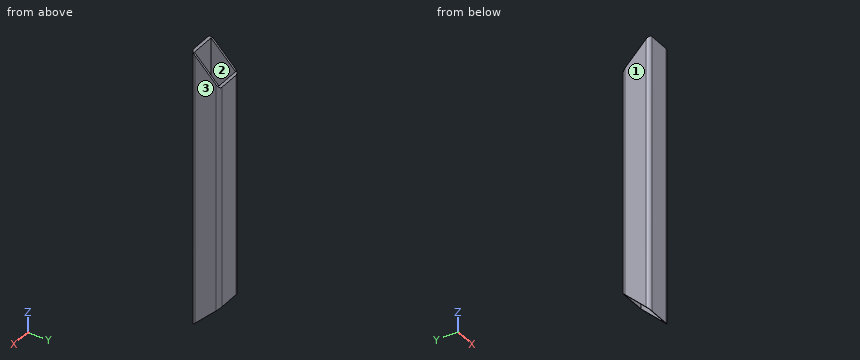
```python
from build123d import *

# Parameters (mm, degrees)
SKETCH1_W           = 50.8
SKETCH1_H           = 50.8
SKETCH1_W_2         = 44.45
SKETCH1_H_2         = 44.45
BOSS_EXTRUDE1_DEPTH = 254
FILLET1_R           = 6.35
CUT_EXTRUDE1_DEPTH  = 914.4


with BuildPart() as part:
    # Sketch1 → Boss-Extrude1 (new, symmetric)
    with BuildSketch(Plane.XY):
        Rectangle(SKETCH1_W, SKETCH1_H)
        Rectangle(SKETCH1_W_2, SKETCH1_H_2, mode=Mode.SUBTRACT)
    extrude(amount=BOSS_EXTRUDE1_DEPTH, both=True)

    # Fillet1
    fillet1_edges = [part.edges().sort_by_distance(p)[0] for p in [
        (-25.4, 25.4, 0),
        (25.4, 25.4, 0),
        (25.4, -25.4, 0),
        (-25.4, -25.4, 0),
    ]]
    fillet(fillet1_edges, radius=FILLET1_R)

    # Sketch2 → Cut-Extrude1 (cut)
    with BuildSketch(Plane.ZY.offset(25.4)):
        Polygon((254, -25.4), (203.2, 25.4), (254, 25.4), align=None)
        Polygon((-254, 25.4), (-254, -25.4), (-203.2, 25.4), align=None)
    extrude(amount=-CUT_EXTRUDE1_DEPTH, mode=Mode.SUBTRACT)


solid = part.part
```
Input: part model. Units: mm. Frame: model coordinates. Face numbers are marked on the shaded views. Give positions to 0.01 mm unless a question says otherwise; leave off trailing zeros. Order: outer loops, then holes, each group sorted by start corner. A loop starts at its lowest first (then second) coordinate and runs counter-clockwise, first axis right, second up. Notation, with made-up numbers: M 63,28.5 L 115,28.5 A22 cw 115,58.5 Z; hole C 12,-22.5 d9. An arc over 180 degrees is marked long. Return JSON: item names as keys, results as strings.
Item 1: Cut plane B-B (x = 9). Return loops of the section in (y, z) (3 decimals).
Solutions:
{"outline": "M -25.4,-254 L -22.225,-250.825 L -22.225,250.825 L -25.4,254 Z; M 22.225,-206.375 L 25.4,-203.2 L 25.4,203.2 L 22.225,206.375 Z"}
Item 2: Cut plane C-C (z = 49). Return loops of the section in (x, y) (3 decimals).
Solutions:
{"outline": "M -25.4,-19.05 A6.35 ccw -19.05,-25.4 L 19.05,-25.4 A6.35 ccw 25.4,-19.05 L 25.4,19.05 A6.35 ccw 19.05,25.4 L -19.05,25.4 A6.35 ccw -25.4,19.05 Z; hole M -22.225,-22.225 L 22.225,-22.225 L 22.225,22.225 L -22.225,22.225 Z"}
Item 3: Ray query, probe 1 along X at (y, z) = (-16.5, 126) (3 decimals); probe 2 along X at (y, z) = (-20, -231) (3 decimals); probe 3 along Y at (x, z) = (19.5, -142.5) (3 decimals). Return the intervals inside material, ascending.
Solutions:
{"probe 1": "-25.4 to -22.225, 22.225 to 25.4", "probe 2": "-25.329 to -22.225, 22.225 to 25.329", "probe 3": "-25.384 to -22.225, 22.225 to 25.384"}
Item 4: Cut plane A-A (y = -12). Return loops of the section in (x, z) (3 decimals), then the cut area to 3 significant figures.
Solutions:
{"outline": "M -25.4,-240.6 L -22.225,-240.6 L -22.225,240.6 L -25.4,240.6 Z; M 22.225,-240.6 L 25.4,-240.6 L 25.4,240.6 L 22.225,240.6 Z", "area": "3,060 mm^2"}
Item 5: Pull-direction query (X, two-part tool) for the marked faces 1, 2 and 3; classes: +X half, -X half, draft (parallel to the pull), parting line (faces both ways), or undercut.
Solutions:
{"face 1": "-X half", "face 2": "undercut", "face 3": "+X half"}
